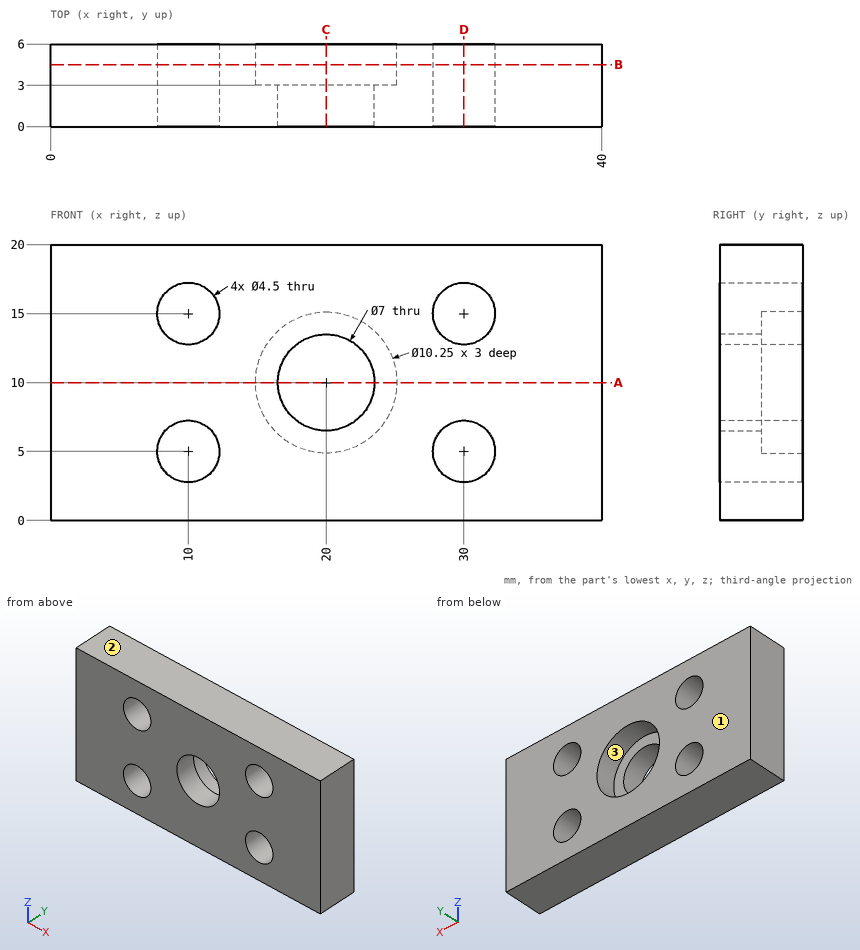
Geometry: see drawing. Coordinates: mm, zero at the bounding-box minimum. Give positions to 0.01 mm unless a question says otherwise; leave off trailing zeros. Loops run counter-clockwise (first coordinate to the right, second up) from the corner with the lowest first, then second, coordinate; pieces in that order, holes last. Notation, with made-up numbers: (23.25, 2) - (45.25, 2) arc R12 ccw to (45.25, 9) - close; hole circle Ø8 at (17.5, -26.5). An arc over 180 degrees is marked (long way). Use CSV: the item, a comma, the result in double quotes. Start each with the question number.
1. Section A-A (z = 10). Output: boundary loops of the cut face in (x, y) (3 decimals).
2. Ray query, L1, parallel to X at y = 1.6, z = 5; L2, parallel to X at y = 5.3, z = 10 (3 decimals); L3, parallel to X at y = 4.55, z = 13.75. Return the intervals inside material, ascending.
3. Section B-B (y = 4.5). Output: boundary loops of the cut face in (x, z) (3 decimals), then the cut area to 3 significant figures.
4. Section D-D (x = 30). Output: boundary loops of the cut face in (y, z), then the cut area to 3 significant figures.
5. Section C-C (x = 20). Output: boundary loops of the cut face in (y, z) (3 decimals).
6. Draft query along Z for the marked faces 1, 2 and 3. Return one class per face: +Z half, -Z half, draft (parallel to the pull), parting line (faces both ways), or undercut.
7. Pin query (flat end, axial travel): pin 1 (5 mm diameter, centred on x = 22.5, z = 7.5, fed in from +Y). Return the tip coordinate at first contact, or that it passes through.
Response:
1,outline,"(0, 0) - (16.5, 0) - (16.5, 3) - (14.875, 3) - (14.875, 6) - (0, 6) - close; (23.5, 0) - (40, 0) - (40, 6) - (25.125, 6) - (25.125, 3) - (23.5, 3) - close"
2,L1,"0 to 7.75, 12.25 to 27.75, 32.25 to 40"
2,L2,"0 to 14.875, 25.125 to 40"
2,L3,"0 to 8.13, 11.87 to 16.51, 23.49 to 28.13, 31.87 to 40"
3,outline,"(0, 0) - (40, 0) - (40, 20) - (0, 20) - close; hole circle Ø4.5 at (10, 5); hole circle Ø4.5 at (10, 15); hole circle Ø10.25 at (20, 10); hole circle Ø4.5 at (30, 5); hole circle Ø4.5 at (30, 15)"
3,area,"654 mm²"
4,outline,"(0, 0) - (6, 0) - (6, 2.75) - (0, 2.75) - close; (0, 7.25) - (6, 7.25) - (6, 12.75) - (0, 12.75) - close; (0, 17.25) - (6, 17.25) - (6, 20) - (0, 20) - close"
4,area,"66.0 mm²"
5,outline,"(0, 0) - (6, 0) - (6, 4.875) - (3, 4.875) - (3, 6.5) - (0, 6.5) - close; (0, 13.5) - (3, 13.5) - (3, 15.125) - (6, 15.125) - (6, 20) - (0, 20) - close"
6,face 1,"draft"
6,face 2,"+Z half"
6,face 3,"undercut"
7,pin 1,"y = 6"
